```python
from build123d import *

# Parameters (mm, degrees)
F0_R     = 10
F1_DEPTH = 25
F2_DEPTH = 50
F3_SIZE  = 2
F4_SIZE  = 2


with BuildPart() as f1:
    # F0 (on Front) → F1 (new body)
    with BuildSketch(Plane.XZ):
        with BuildLine():
            ThreePointArc((2.083333, -24.913043), (18.399502, -16.92508), (25, 0))
            ThreePointArc((25, 0), (18.399502, 16.92508), (2.083333, 24.913043))
            ThreePointArc((2.083333, 24.913043), (-25, 0), (2.083333, -24.913043))
        make_face()
        Circle(F0_R, mode=Mode.SUBTRACT)
        with BuildLine():
            ThreePointArc((2.083333, 24.913043), (18.399502, 16.92508), (25, 0))
            ThreePointArc((25, 0), (18.399502, -16.92508), (2.083333, -24.913043))
            Line((2.083333, -24.913043), (91.458333, -17.43913))
            ThreePointArc((91.458333, -17.43913), (72.5, 0), (91.458333, 17.43913))
            Line((91.458333, 17.43913), (2.083333, 24.913043))
        make_face()
        with BuildLine():
            ThreePointArc((107.5, 0), (102.879651, 11.847556), (91.458333, 17.43913))
            ThreePointArc((91.458333, 17.43913), (72.5, 0), (91.458333, -17.43913))
            ThreePointArc((91.458333, -17.43913), (102.879651, -11.847556), (107.5, 0))
        make_face()
        with Locations((90, 0)):
            Circle(F0_R, mode=Mode.SUBTRACT)
    extrude(amount=F1_DEPTH)

    # F0 (on Front) → F2 (join)
    with BuildSketch(Plane.XZ):
        with BuildLine():
            ThreePointArc((2.083333, -24.913043), (18.399502, -16.92508), (25, 0))
            ThreePointArc((25, 0), (18.399502, 16.92508), (2.083333, 24.913043))
            ThreePointArc((2.083333, 24.913043), (-25, 0), (2.083333, -24.913043))
        make_face()
        Circle(F0_R, mode=Mode.SUBTRACT)
    extrude(amount=F2_DEPTH)

    # F3
    f3_edges = [f1.edges().sort_by_distance(p)[0] for p in [
        (-2.083333, -50, 24.913043),
        (-10, -50, 0),
        (80, -25, 0),
    ]]
    chamfer(f3_edges, length=F3_SIZE)

    # F4
    f4_edges = [f1.edges().sort_by_distance(p)[0] for p in [
        (-10, 0, 0),
        (80, 0, 0),
    ]]
    chamfer(f4_edges, length=F4_SIZE)


solid = f1.part
```
Check sheet for the modelled part. Datum: model origin and axes. Units: mm. Give positions to 0.01 mm unless a question says otherwise; leave off trailing zeros. Order: outer loops, then holes, each group sorted by start corner. A loop starts at its lowest first (then second) coordinate and runs counter-clockwise, first axis right, second up. Notation, with made-up numbers: M 64.5,35 L 102.5,35 A17 ccw 102.5,54 Z; hole C 79.5,89.25 d3. An arc over 180 degrees is marked long. Answer in a Markdown table with one row per item.
1) Thickness scan on L1, parallel to Z at x = 0, y = -17.5; L2, parallel to Y at x = 67, z = -3.5; L3, parallel to Z at x = 90, y = -9. Record the ranges inside material, lowest first. Write a range as [from, to].
Filled sheet:
| item | result |
|---|---|
| L1 | z = [-25, -10], [10, 25] |
| L2 | y = [-25, 0] |
| L3 | z = [-17.56, -10], [10, 17.56] |
2) Cross-section at B-B, the plane x = 0. Enter the section's corners in (y, z), plus the area to 3 significant figures.
Filled sheet:
| item | result |
|---|---|
| outline | M -50,-23 L -48,-25 L 0,-25 L 0,-12 L -2,-10 L -48,-10 L -50,-12 Z; M -50,12 L -48,10 L -2,10 L 0,12 L 0,25 L -48,25 L -50,23 Z |
| area | 1,490 mm2 |
3) Gauge pin test, flat ends, axial feed: P1, Ø1, axis at y = -32.5, z = 14.5, coming from the -X side; P2, Ø1.5, axis at x = 54, y = -14, coming from the -Z side; P3, Ø16, axis at x = 90, z = 0, coming from the +Y side; P4, Ø12, axis at x = 58.5, z = -10, coming from the -Y side. Record the tip position at first contact, or that the pin passes through.
Filled sheet:
| item | result |
|---|---|
| P1 | stops at x = -20.71 |
| P2 | stops at z = -20.63 |
| P3 | passes through |
| P4 | stops at y = -25 |
4) Cross-section at C-C, the plane x = 90. Enter the section's corners in (y, z), plus the area to 3 significant figures.
Filled sheet:
| item | result |
|---|---|
| outline | M -25,-17.56 L 0,-17.56 L 0,-12 L -2,-10 L -23,-10 L -25,-12 Z; M -25,12 L -23,10 L -2,10 L 0,12 L 0,17.56 L -25,17.56 Z |
| area | 370 mm2 |
5) Cross-section at A-A, the plane y = -19. Enter the section's corners in (x, z).
Filled sheet:
| item | result |
|---|---|
| outline | M 2.08,-24.91 L 91.46,-17.44 A17.5 ccw 91.46,17.44 L 2.08,24.91 A25 ccw long Z; hole C 0,0 d20; hole C 90,0 d20 |
6) Release check for a two-part mould opening along X. For faces 1 (the flat face through (46.15, -12.32, -21.23)), 2 (the conical face through (81.965, -23.125, -6.161)), 3 (the flat face through (40, 0, 0)) record: +X half, -X half, draft (parallel to the pull), parting line (faces both ways), or undercut.
Filled sheet:
| item | result |
|---|---|
| face 1 | +X half |
| face 2 | undercut |
| face 3 | draft |
7) Cross-section at D-D, the plane z = 7. Count the separate pieces of the cut face and the enclosed holes in it, plus the area to 3 significant figures.
Filled sheet:
| item | result |
|---|---|
| separate pieces | 3 |
| enclosed holes | 0 |
| area | 3,350 mm2 |
